Could you check a few things on this model? Use its own coordinates, in mm. A direction names the side the tool comes from. Coordinates: 2 decimals unless noted, no trailing zeros. Loops run counter-clockwise (first coordinate to the right, second up) from the corner with the lowest first, then second, coordinate; pieces in that order, holes last. Notation, with made-up numbers: (41, 74.5) -> (69, 74.5) arc R23 ccw to (69, 83.5) -> close; hole circle Ø8 at (5.5, -0.75). An arc over 180 degrees is marked (long way). One line per question, with ' | ' between items.
from build123d import *

# Parameters (mm, degrees)
BOSS_EXTRUDE1_DEPTH                            = 25.4
SKETCH2_R                                      = 3.96875
CUT_EXTRUDE1_DEPTH                             = 4.175
CSK_FOR_2_FLAT_HEAD_MACHINE_SCREW1_D           = 2.4384
CSK_FOR_2_FLAT_HEAD_MACHINE_SCREW1_CSINK_D     = 4.3688
CSK_FOR_2_FLAT_HEAD_MACHINE_SCREW1_CSINK_ANGLE = 82


with BuildPart() as part:
    # Sketch1 → Boss-Extrude1 (new body)
    with BuildSketch(Plane(origin=(0, 0, 0), x_dir=(1, 0, 0), z_dir=(0, 1, 0))):
        Polygon((0, 0), (0, 44.45), (3.175, 44.45), (3.175, 3.175), (25.4, 3.175), (25.4, 0), align=None)
    extrude(amount=BOSS_EXTRUDE1_DEPTH)

    # Sketch2 → Cut-Extrude1 (cut, through all)
    with BuildSketch(Plane(origin=(3.175, 0, 0), x_dir=(0, 0, -1), z_dir=(1, 0, 0))):
        with Locations((31.75, 12.7)):
            Circle(SKETCH2_R)
    extrude(amount=-CUT_EXTRUDE1_DEPTH, mode=Mode.SUBTRACT)

    # CSK for #2 Flat Head Machine Screw1 (through all)
    with Locations(Plane(origin=(0, 0, -3.175), x_dir=(-1, 0, 0), z_dir=(0, 0, -1))):
        with Locations((-14.2875, 19.05), (-14.2875, 6.35)):
            CounterSinkHole(CSK_FOR_2_FLAT_HEAD_MACHINE_SCREW1_D / 2, CSK_FOR_2_FLAT_HEAD_MACHINE_SCREW1_CSINK_D / 2, counter_sink_angle=CSK_FOR_2_FLAT_HEAD_MACHINE_SCREW1_CSINK_ANGLE)


solid = part.part
1) If we section it at D-D on y = 12.7: Please give me the cut outline in (x, z) (3 decimals), and give its area (3 significant figures).
Data:
outline: (0, -44.45) -> (3.175, -44.45) -> (3.175, -35.719) -> (0, -35.719) -> close; (0, -27.781) -> (3.175, -27.781) -> (3.175, -3.175) -> (25.4, -3.175) -> (25.4, 0) -> (0, 0) -> close | area: 186 mm²
2) On a 3-axis mill with a long thin cutter (end or side, diameter ignored), from which of +Z, -Z, +X, -X, +Y, -Y can I reach the whole of each face in a straight line? I mean faces 5 (the face through (2, 13, -44.45)), 6 (the face through (14, 13, -3.175)). Say none if no direction works.
Data:
face 5: -Z, +X, -X, +Y, -Y | face 6: -Z, +X, +Y, -Y
3) If we section it at C-C on x = 2: Please give me the cut outline in (y, z).
Data:
outline: (0, -44.45) -> (25.4, -44.45) -> (25.4, 0) -> (0, 0) -> close; hole circle Ø7.94 at (12.7, -31.75)
4) If we section it at B-B on z = -31.75: Please give me the cut outline in (x, y) (3 decimals), and give its area (3 significant figures).
Data:
outline: (0, 0) -> (3.175, 0) -> (3.175, 8.731) -> (0, 8.731) -> close; (0, 16.669) -> (3.175, 16.669) -> (3.175, 25.4) -> (0, 25.4) -> close | area: 55.4 mm²
5) I'm going to push flat-ended pins straight in: pin 1 Ø10 at (y, z) = (8, -27.5) entering from +X (3 decimals); pin 2 Ø1 at (x, y) = (13.5, 18) entering from -Z; pin 3 Ø11 at (x, y) = (9.5, 17.5) entering from -Z (3 decimals). Where does each tip first touch, or does it pass through?
Data:
pin 1: x = 3.175 | pin 2: z = -2.75 | pin 3: z = -3.175
6) We'd pull the mould along Y, two halves only. Please class faces 1 (the face through (3.175, 13, -24)), 2 (the face through (2, 0, -14)), 3 (the face through (2, 25.4, -14)), 4 (the face through (15.414, 5.883, -1.018)): pulls with the +Y half, pulls with the -Y half, needs draft (parallel to the pull), parting line crosses it, or undercut.
Data:
face 1: needs draft | face 2: pulls with the -Y half | face 3: pulls with the +Y half | face 4: undercut
7) If we section it at A-A on y = 19.05: Please give me the cut outline in (x, z) (3 decimals).
Data:
outline: (0, -44.45) -> (3.175, -44.45) -> (3.175, -3.175) -> (12.103, -3.175) -> (13.068, -2.065) -> (13.068, 0) -> (0, 0) -> close; (15.507, -2.065) -> (16.472, -3.175) -> (25.4, -3.175) -> (25.4, 0) -> (15.507, 0) -> close
8) I need wall thicknesses on line 1 along X through (y, z) = (19.05, -1.6); line 2 along Y through (x, z) = (1.05, -31.75); line 3 along Z through (x, y) = (19.5, 24.5) (3 decimals). Which ranges of each line are inside material? Lowest first, please. Write a range as from..to.
Data:
line 1: 0..13.07, 15.51..25.4 | line 2: 0..8.73, 16.67..25.4 | line 3: -3.175..0
